Study the drawing (mm; zero at the part's minimum x, y, z) and answer. Give positions to 0.01 mm unless a question says otherwise; leave off trailing zeros. Order: outer loops, then holes, each group sorted by start corner. A loop starts at its lowest first (then second) coordinate and runs counter-clockwise, first axis right, second up.
Item 1: A cutting plane is placed at A-A (x = 90). Write down the section's boundary in (y, z), plus the area to 3 significant figures.
Item 2: Given pin 1 Ø5 at (y, z) = (91.5, 494) entering from +X; pin 2 Ø5 at (x, y) = (123.5, 106) entering from +Z; pin 3 Ø4 at (x, y) = (32, 82.5) entering from -Z, each flat-ended and moving along its own axis, determine where each tip first touches the part or whether it passes through.
Item 3: Find the intervals of material crossed by line 1 along Y through (x, z) = (90, 22); line 2 along Z through (x, y) = (165, 50.5); line 3 along Z through (x, y) = (157, 75), in increasing order.
Item 4: A cutting plane is placed at D-D (x = 154.5). Write down the section's boundary in (y, z).
Item 5: The mould has two halves that part along X. Classify the marked faces 1, 2 and 3: +X half, -X half, draft (parallel to the pull), parting line (faces both ways), or undercut.
Item 6: A cutting plane is placed at C-C (z = 431.5). Write down the section's boundary in (x, y), plus the area to 3 significant figures.
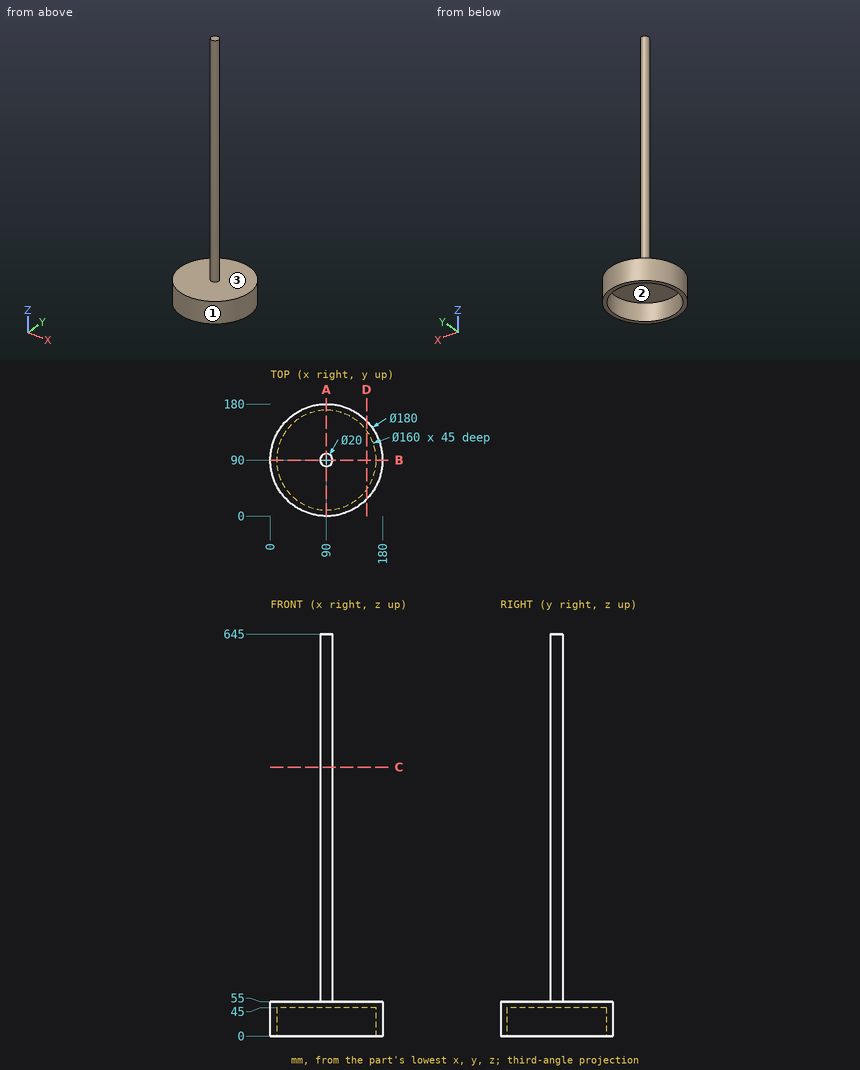
Response values:
1. outline: (0, 0) - (10, 0) - (10, 45) - (170, 45) - (170, 0) - (180, 0) - (180, 55) - (100, 55) - (100, 645) - (80, 645) - (80, 55) - (0, 55) - close
1. area: 14,500 mm2
2. pin 1: stops at x = 100
2. pin 2: stops at z = 55
2. pin 3: stops at z = 45
3. line 1: y = 0 to 10, 170 to 180
3. line 2: z = 0 to 55
3. line 3: z = 45 to 55
4. outline: (27.23, 0) - (42.67, 0) - (42.67, 45) - (137.33, 45) - (137.33, 0) - (152.77, 0) - (152.77, 55) - (27.23, 55) - close
5. face 1: parting line
5. face 2: undercut
5. face 3: draft
6. outline: circle Ø20 at (90, 90)
6. area: 314 mm2
